Work out the finished part from the listing and answer in its coordinate system (mm). Give positions to 0.01 mm unless a question says otherwise; leave off trailing zeros. Write each loop counter-clockwise with the first axis right and the second up, starting at its lowest first coordinate (ties: lowest second). Pieces come first, ordered by that corner, then holes. Notation, with made-up numbers: (21.5, -14) -> (67.5, -14) arc R13 ccw to (67.5, 4) -> close; hole circle Ø6 at (81.5, -20.5). An arc over 180 degrees is marked (long way). Write item = value, one per line. Start each with the question number.
from build123d import *

# Parameters (mm, degrees)
ESQUISSE1_W        = 70
ESQUISSE1_H        = 58.15
ESQUISSE1_R        = 1.95
ESQUISSE1_R_2      = 1
ESQUISSE1_R_3      = 2.640146182
ESQUISSE1_W_2      = 7
ESQUISSE1_H_2      = 5.5
ESQUISSE1_W_3      = 3.5
ESQUISSE1_H_3      = 4
BOSS_EXTRU_1_DEPTH = 5
ESQUISSE2_R        = 9.1
CR_NEAUX_DEPTH     = 5
ESQUISSE3_W        = 20
ESQUISSE3_H        = 7.07
ESQUISSE3_W_2      = 5
ESQUISSE3_H_2      = 15
ESQUISSE3_H_3      = 10
CR_NEAUX_2_DEPTH   = 5


with BuildPart() as part:
    # Esquisse1 → Boss.-Extru.1 (new body)
    with BuildSketch(Plane.XY):
        with Locations((35, 29.075)):
            Rectangle(ESQUISSE1_W, ESQUISSE1_H)
        with Locations((12.149282213, 31.8)):
            Circle(ESQUISSE1_R, mode=Mode.SUBTRACT)
        with Locations((4.649282213, 27.7)):
            Circle(ESQUISSE1_R_2, mode=Mode.SUBTRACT)
        with Locations((14.749282213, 16.45)):
            Circle(ESQUISSE1_R_2, mode=Mode.SUBTRACT)
        with Locations((34.649282213, 16.45)):
            Circle(ESQUISSE1_R_2, mode=Mode.SUBTRACT)
        with Locations((54.549282213, 16.45)):
            Circle(ESQUISSE1_R_2, mode=Mode.SUBTRACT)
        with Locations((64.649282213, 27.7)):
            Circle(ESQUISSE1_R_2, mode=Mode.SUBTRACT)
        with Locations((54.654459148, 36.574348259)):
            Circle(ESQUISSE1_R_3, mode=Mode.SUBTRACT)
        with Locations((14.644105278, 36.574348259)):
            Circle(ESQUISSE1_R_3, mode=Mode.SUBTRACT)
        with BuildLine():
            Line((26.249282245, 52.35), (43.049282245, 52.35))
            Line((43.049282245, 52.35), (43.049282245, 45.7))
            Line((43.049282245, 45.7), (43.649282213, 45.7))
            ThreePointArc((43.649282213, 45.7), (45.349282213, 44), (43.649282213, 42.3))
            Line((43.649282213, 42.3), (43.049282218, 42.3))
            Line((43.049282218, 42.3), (43.049282218, 35.65))
            Line((43.049282218, 35.65), (42.149282213, 35.65))
            Line((42.149282213, 35.65), (42.149282213, 28.2))
            Line((42.149282213, 28.2), (39.649282213, 28.2))
            Line((39.649282213, 28.2), (39.649282213, 35.65))
            Line((39.649282213, 35.65), (30.649282213, 35.65))
            Line((30.649282213, 35.65), (30.649282213, 27.8))
            Line((30.649282213, 27.8), (25.149282213, 27.8))
            Line((25.149282213, 27.8), (25.149282213, 23.3))
            Line((25.149282213, 23.3), (21.149282213, 23.3))
            Line((21.149282213, 23.3), (21.149282213, 33.3))
            Line((21.149282213, 33.3), (25.649282213, 33.3))
            Line((25.649282213, 33.3), (25.649282213, 36.5))
            Line((25.649282213, 36.5), (20.449282213, 36.5))
            Line((20.449282213, 36.5), (20.449282213, 42.5))
            Line((20.449282213, 42.5), (24.849282213, 42.5))
            ThreePointArc((24.849282213, 42.5), (24.000039995, 44.412310574), (25.64928225, 45.7))
            Line((25.64928225, 45.7), (26.249282245, 45.7))
            Line((26.249282245, 45.7), (26.249282245, 52.35))
        make_face(mode=Mode.SUBTRACT)
        with Locations((13.149282213, 24.55)):
            Rectangle(ESQUISSE1_W_2, ESQUISSE1_H_2, mode=Mode.SUBTRACT)
        with BuildLine():
            Line((6.557160615, 18), (9.649282213, 18))
            Line((9.649282213, 18), (9.649282213, 13.7))
            Line((9.649282213, 13.7), (6.770602556, 13.7))
            ThreePointArc((6.770602556, 13.7), (1.702909759, 15.603748964), (6.557160615, 18))
        make_face(mode=Mode.SUBTRACT)
        with BuildLine():
            Line((22.649282213, 17.918524844), (22.649282213, 18.4))
            Line((22.649282213, 18.4), (18.649282213, 18.4))
            Line((18.649282213, 18.4), (18.649282213, 14.1))
            Line((18.649282213, 14.1), (22.20387836, 14.1))
            ThreePointArc((22.20387836, 14.1), (27.579416484, 15.40822061), (22.649282213, 17.918524844))
        make_face(mode=Mode.SUBTRACT)
        with BuildLine():
            Line((42.139302133, 17.3), (39.649282213, 17.3))
            Line((39.649282213, 17.3), (39.649282213, 14.8))
            Line((39.649282213, 14.8), (41.856434204, 14.8))
            ThreePointArc((41.856434204, 14.8), (44.004893082, 12.87123939), (46.770602556, 13.7))
            Line((46.770602556, 13.7), (50.649282213, 13.7))
            Line((50.649282213, 13.7), (50.649282213, 18.3))
            Line((50.649282213, 18.3), (47.149282213, 18.3))
            Line((47.149282213, 18.3), (47.149282213, 17.316045976))
            ThreePointArc((47.149282213, 17.316045976), (44.639833994, 18.69998487), (42.139302133, 17.3))
        make_face(mode=Mode.SUBTRACT)
        with Locations((54.399282213, 23.3)):
            Rectangle(ESQUISSE1_W_3, ESQUISSE1_H_3, mode=Mode.SUBTRACT)
        with BuildLine():
            Line((58.649282213, 30.554006421), (58.649282213, 29.8))
            Line((58.649282213, 29.8), (61.649282213, 29.8))
            Line((61.649282213, 29.8), (61.649282213, 31.3))
            Line((61.649282213, 31.3), (59.034089895, 31.3))
            ThreePointArc((59.034089895, 31.3), (55.416262488, 32.69394778), (58.649282213, 30.554006421))
        make_face(mode=Mode.SUBTRACT)
        with BuildLine():
            Line((63.149282213, 19.3), (63.149282213, 18.290177159))
            ThreePointArc((63.149282213, 18.290177159), (67.498784507, 14.986562594), (62.080235697, 14.3))
            Line((62.080235697, 14.3), (58.649282213, 14.3))
            Line((58.649282213, 14.3), (58.649282213, 19.3))
            Line((58.649282213, 19.3), (63.149282213, 19.3))
        make_face(mode=Mode.SUBTRACT)
    extrude(amount=BOSS_EXTRU_1_DEPTH)

    # Esquisse2 → Cr_neaux (cut)
    with BuildSketch(Plane.XY.offset(5)):
        with Locations((35, 44)):
            Circle(ESQUISSE2_R)
    extrude(amount=-CR_NEAUX_DEPTH, mode=Mode.SUBTRACT)

    # Esquisse3 → Cr_neaux 2 (add)
    with BuildSketch(Plane.XY.offset(5)):
        with Locations((35, 61.685)):
            Rectangle(ESQUISSE3_W, ESQUISSE3_H)
        with Locations((2.5, 61.685)):
            Rectangle(ESQUISSE3_W_2, ESQUISSE3_H)
        with Locations((-2.5, 15.75)):
            Rectangle(ESQUISSE3_W_2, ESQUISSE3_H_2)
        with Locations((-2.5, 43.15)):
            Rectangle(ESQUISSE3_W_2, ESQUISSE3_H_3)
        with Locations((72.5, 43.15)):
            Rectangle(ESQUISSE3_W_2, ESQUISSE3_H_3)
        with Locations((72.5, 15.75)):
            Rectangle(ESQUISSE3_W_2, ESQUISSE3_H_2)
        with Locations((67.5, 61.685)):
            Rectangle(ESQUISSE3_W_2, ESQUISSE3_H)
    extrude(amount=-CR_NEAUX_2_DEPTH)


solid = part.part
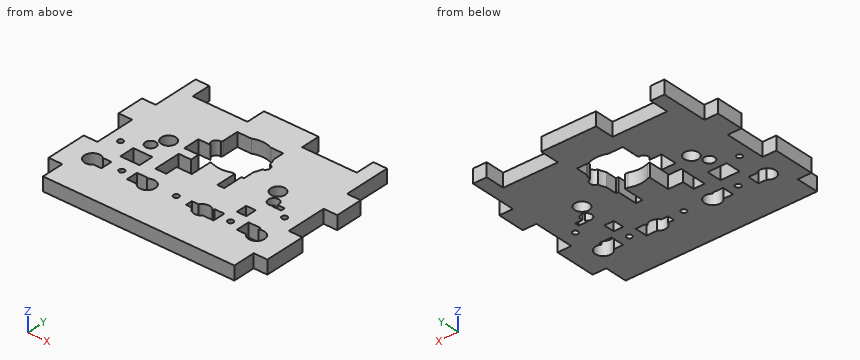
(1) A cutting plane is placed at C-C, the plane y = 55. Write down the section's boundary in (x, z), then the cut area to 3 significant figures.
(2) A cutting plane is placed at B-B, the plane y = 16.45. State how many separate pieces and enclosed holes the cut face has, then the cut area to 3 significant figures.
(3) Find the intervals of material crossed by line 1 along Y through (x, z) = (40.5, 0.8); line 2 along X through (y, z) = (39.5, 0.6); line 3 along Y through (x, z) = (4.5, 2.15), in increasing order.
(4) Each of these flat-tipped pins is pushed along its axis until it touches: pin 1 (1.3 mm diameter, centred on y = 25.5, z = 3, fed in from -X); pin 2 (1.5 mm diameter, centred on y = 26, z = 2.5, fed in from +X); pin 3 (1.5 mm diameter, centred on x = 15, z = 1.5, fed in from +Y). Where does it stop, or does it pass through?
(5) A cutting plane is placed at A-A, the plane x = 48.5. Write down the section's boundary in (y, z), then the cut area to 3 significant figures.
Results list:
q1.outline = (0, 0) -> (70, 0) -> (70, 5) -> (0, 5) -> close
q1.area = 350 mm²
q2.separate_pieces = 8
q2.enclosed_holes = 0
q2.area = 187 mm²
q3.line_1 = 0 to 14.8, 17.3 to 28.2, 52.35 to 65.22
q3.line_2 = -5 to 20.45, 43.05 to 75
q3.line_3 = 0 to 12.8, 18.7 to 26.71, 28.69 to 65.22
q4.pin_1 = 0
q4.pin_2 = 70
q4.pin_3 = 58.15
q5.outline = (0, 0) -> (13.7, 0) -> (13.7, 5) -> (0, 5) -> close; (18.3, 0) -> (58.15, 0) -> (58.15, 5) -> (18.3, 5) -> close
q5.area = 268 mm²
